For this review, take the finished solid that the model builds, in its own axes (mm). Round coordinates to 2 decimals unless told otherwise and drop trailing zeros. Order: outer loops, then holes, each group sorted by start corner. A loop starts at its lowest first (then second) coordinate and runs counter-clockwise, first axis right, second up.
Autodesk Inventor part; units mm, degrees
ref_plane "YZ Plane" through (0, 0, 0) normal (1, 0, 0) x (0, 1, 0)
ref_plane "XZ Plane" through (0, 0, 0) normal (0, 1, 0) x (-1, 0, 0)
ref_plane "XY Plane" through (0, 0, 0) normal (0, 0, 1) x (1, 0, 0)
sketch "Sketch1" plane through (0, 0, 0) normal (0, 0, 1) x (1, 0, 0)
  line L0 (0, 0) -> (362.9152, 0)
  line L1 (362.9152, 0) -> (362.9152, 127)
  line L2 (362.9152, 127) -> (0, 127)
  line L3 (0, 127) -> (0, 0)
  dimension "d0" = 362.9152
  dimension "d1" = 127
extrude "Extrusion1" add sketch "Sketch1" along normal blind 3.175
sketch "Sketch2" plane through (0, 0, 3.175) normal (0, 0, 1) x (1, 0, 0)
  line L0 (0, 127) -> (0, 0)
  line L1 (362.9152, 0) -> (362.9152, 127)
  line L2 (362.9152, 127) -> (0, 127)
  line L3 (0, 0) -> (362.9152, 0)
  point P0 (12.7, 25.4)
  point P1 (12.7, 63.5)
  point P2 (350.2152, 25.4)
  point P3 (350.2152, 63.5)
  point P4 (12.7, 101.6)
  point P5 (350.2152, 101.6)
  dimension "d4" = 12.7
  dimension "d5" = 12.7
  dimension "d6" = 12.7
  dimension "d7" = 12.7
  dimension "d8" = 12.7
  dimension "d9" = 12.7
  dimension "d10" = 25.4
  dimension "d11" = 25.4
  dimension "d12" = 38.1
hole "Hole1" at (12.7, 25.4, 3.175) at (12.7, 63.5, 3.175) at (350.2152, 25.4, 3.175) at (350.2152, 63.5, 3.175) at (12.7, 101.6, 3.175) at (350.2152, 101.6, 3.175) direction (0, 0, -1) diameter 4.8514 end through all
sketch "Sketch3" plane through (0, 0, 3.175) normal (0, 0, 1) x (1, 0, 0)
  line L0 (0, 127) -> (0, 0)
  line L1 (362.9152, 0) -> (362.9152, 127)
  line L2 (0, 127) -> (362.9152, 127)
  line L3 (362.9152, 127) -> (362.9152, 82.55)
  line L4 (362.9152, 82.55) -> (0, 82.55)
  line L5 (0, 82.55) -> (0, 127)
  line L6 (0, 0) -> (362.9152, 0)
  line L7 (91.1104, 0) -> (300.3978, 0)
  line L8 (300.3978, 0) -> (300.3978, -76.2)
  line L9 (300.3978, -76.2) -> (91.1104, -76.2)
  line L10 (91.1104, -76.2) -> (91.1104, 0)
  dimension "d20" = 76.2
  dimension "d21" = 44.45
extrude "Extrusion2" cut sketch "Sketch3" against normal blind 25.4 contours L2 L1 L4 L0
sketch "Sketch4" plane through (0, 0, 3.175) normal (0, 0, 1) x (1, 0, 0)
  line L0 (0, 0) -> (362.9152, 0)
  line L1 (76.2, 0) -> (286.7152, 0)
  line L2 (286.7152, 0) -> (286.7152, -76.2)
  line L3 (286.7152, -76.2) -> (76.2, -76.2)
  line L4 (76.2, -76.2) -> (76.2, 0)
  line L5 (0, 82.55) -> (0, 0)
  line L6 (362.9152, 0) -> (362.9152, 82.55)
  dimension "d24" = 76.2
  dimension "d25" = 76.2
  dimension "d26" = 76.2
extrude "Extrusion3" add sketch "Sketch4" against normal blind 3.175
sketch "Sketch5" plane through (0, 0, 3.175) normal (0, 0, 1) x (1, 0, 0)
  line L0 (286.7152, -76.2) -> (76.2, -76.2)
  line L1 (76.2, -76.2) -> (76.2, 0)
  point P0 (0, 0)
  point P1 (105.2576, -63.5)
  point P2 (143.3576, -63.5)
  point P3 (181.4576, -63.5)
  point P4 (219.5576, -63.5)
  point P5 (257.6576, -63.5)
  dimension "d29" = 38.1
  dimension "d30" = 38.1
  dimension "d31" = 38.1
  dimension "d32" = 38.1
  dimension "d33" = 12.7
  dimension "d34" = 29.0576
hole "Hole2" at (105.2576, -63.5, 3.175) at (143.3576, -63.5, 3.175) at (181.4576, -63.5, 3.175) at (219.5576, -63.5, 3.175) at (257.6576, -63.5, 3.175) direction (0, 0, -1) diameter 4.8514 end through all
properties part number "SUP_021_LexanShield"
(1) Add section B-B on y = -52.5. Give the boundary of the cut face in (x, z) (3 decimals), plus the area to 3 significant figures.
(2) Add section C-C on x = 24. Give the boundary of the cut face in (y, z) (3 decimals).
(3) Wall thickness on L1, parallel to X at y = -63.5, z = 2.5; L2, parallel to X at y = 25.4, z = 2.5; L3, parallel to X at y = 24, z = 0.25: over which ranges is each line inside the solid? List them lowest first.
(4) Clearance check with flat-ended pins moving along their axes: P1, Ø1.6, axis at y = -49.5, z = 1, coming from the -X side; P2, Ø4, axis at x = 12.7, y = 63.5, coming from the -Z side; P3, Ø1, axis at y = -22.5, z = 1.5, coming from the +X side. State where each tip first meets the part, or that it passes through.
(5) Add section A-A on z = 2.2. Count the separate pieces of the cut face and the enclosed holes in it, plus the area to 3 significant figures.
Here are the results:
1. outline: (76.2, 0) - (286.715, 0) - (286.715, 3.175) - (76.2, 3.175) - close
1. area: 668 mm2
2. outline: (0, 0) - (82.55, 0) - (82.55, 3.175) - (0, 3.175) - close
3. L1: x = 76.2 to 102.83, 107.68 to 140.93, 145.78 to 179.03, 183.88 to 217.13, 221.98 to 255.23, 260.08 to 286.72
3. L2: x = 0 to 10.27, 15.13 to 347.79, 352.64 to 362.92
3. L3: x = 0 to 10.72, 14.68 to 348.23, 352.2 to 362.92
4. P1: stops at x = 76.2
4. P2: passes through
4. P3: stops at x = 286.72
5. separate pieces: 1
5. enclosed holes: 9
5. area: 45,800 mm2
